from build123d import *

# Parameters (mm, degrees)
SKETCH2_R           = 4.195
SKETCH2_R_2         = 10.305
BOSS_EXTRUDE1_DEPTH = 5.96
FILLET1_R           = 1
SKETCH3_R           = 13.8
SKETCH3_R_2         = 10.305
BOSS_EXTRUDE2_DEPTH = 3.15
FILLET2_R           = 1


with BuildPart() as part:
    # Sketch2 → Boss-Extrude1 (new body)
    with BuildSketch(Plane.XY):
        with BuildLine():
            Line((101.69, 0), (101.69, 15.7))
            ThreePointArc((101.69, 15.7), (97.091576465, 26.801576465), (85.99, 31.4))
            Line((85.99, 31.4), (0, 31.4))
            ThreePointArc((0, 31.4), (-11.101576465, 26.801576465), (-15.7, 15.7))
            ThreePointArc((-15.7, 15.7), (-11.101576465, 4.598423535), (0, 0))
            Line((0, 0), (22.15, 0))
            Line((22.15, 0), (55.695, -63.695))
            ThreePointArc((55.695, -63.695), (58.476021113, -70.408978887), (65.19, -73.19))
            ThreePointArc((65.19, -73.19), (71.903978887, -70.408978887), (74.685, -63.695))
            ThreePointArc((74.685, -63.695), (74.678632674, -63.462256539), (74.673581437, -63.229480796))
            ThreePointArc((74.673581437, -63.229480796), (79.11133413, -43.842864153), (92.1177, -28.7973))
            ThreePointArc((92.1177, -28.7973), (98.886338242, -25.993638242), (101.69, -19.225))
            Line((101.69, -19.225), (101.69, -12.489796776))
            Line((101.69, -12.489796776), (101.69, 0))
        make_face()
        with BuildLine():
            ThreePointArc((69.385, -63.695), (68.156312947, -66.661312947), (65.19, -67.89))
            ThreePointArc((65.19, -67.89), (62.223687053, -60.728687053), (69.385, -63.695))
        make_face(mode=Mode.SUBTRACT)
        with BuildLine():
            ThreePointArc((1.34, 8.01), (-4.097651147, 10.262348853), (-6.35, 15.7))
            ThreePointArc((-6.35, 15.7), (-4.097651147, 21.137651147), (1.34, 23.39))
            Line((1.34, 23.39), (44.31, 23.39))
            ThreePointArc((44.31, 23.39), (52, 15.7), (44.31, 8.01))
            Line((44.31, 8.01), (1.34, 8.01))
        make_face(mode=Mode.SUBTRACT)
        with Locations((92.1177, -19.225)):
            Circle(SKETCH2_R, mode=Mode.SUBTRACT)
        with Locations((85.99, 15.7)):
            Circle(SKETCH2_R_2, mode=Mode.SUBTRACT)
    extrude(amount=BOSS_EXTRUDE1_DEPTH)

    # Fillet1
    fillet1_edges = [part.edges().sort_by_distance(p)[0] for p in [
        (92.1177, -28.7973, 2.98),
        (55.695, -63.695, 2.98),
        (22.15, 0, 2.98),
    ]]
    fillet(fillet1_edges, radius=FILLET1_R)

    # Sketch3 → Boss-Extrude2 (add)
    with BuildSketch(Plane.XY.offset(5.96)):
        with Locations((85.99, 15.7)):
            Circle(SKETCH3_R)
        with Locations((85.99, 15.7)):
            Circle(SKETCH3_R_2, mode=Mode.SUBTRACT)
    extrude(amount=BOSS_EXTRUDE2_DEPTH)

    # Fillet2
    fillet2_edges = [part.edges().sort_by_distance(p)[0] for p in [
        (72.19, 15.7, 9.11),
        (75.685, 15.7, 9.11),
    ]]
    fillet(fillet2_edges, radius=FILLET2_R)


solid = part.part
Source: CAD feature listing. Evaluate the final solid. Frame: model axes, mm. A direction names the side the tool comes from. Give positions to 0.01 mm unless a question says otherwise; leave off trailing zeros. Write each loop counter-clockwise with the first axis right and the second up, starting at its lowest first coordinate (ties: lowest second). Pieces come first, ordered by that corner, then holes. Notation, with made-up numbers: M 80,68.5 L 109,68.5 A18 cw 109,96.5 Z; hole C -20,8 d6. An arc over 180 degrees is marked long. Return JSON: item names as keys, results as strings. Group by question number.
1) First-contact query: pin 1 Ø12 at (x, y) = (59, -50.5) entering from +Z; pin 2 Ø3 at (x, z) = (33.5, 2) entering from -Y; pin 3 Ø1.8 at (x, z) = (7, 3) entering from -Y. Flat tips, straight axial feed; report the tip coordinate or a pass-through.
2) Cut plane B-B, the plane y = -20.5. Output: boundary loops of the cut face in (x, z), then the cut area to 3 significant figures.
3) Set-up query: faces 1 (the face through (11, 0, 3)), 2 (the face through (23, 8.01, 3)), 3 (the face through (93.409, 27.336, 7.02)), 4 (the face through (98.92, -25.96, 2.94)). Return all of +Z, -Z, +X, -X, +Y, -Y with unobstructed straight access to the full face (end or side cutting, diameter ignored); none if empty.
4) Cut plane A-A, the plane x = 18.5. Output: boundary loops of the cut face in (y, z), then the cut area to 3 significant figures.
5) Cut plane C-C, the plane z = 1.75. Give the number of separate pieces and of enclosed holes in the cut face, then the cut area to 3 significant figures.
6) Draft query along Y for faces 5 (the face through (38.775, -31.567, 2.938)), 6 (the face through (55, -9, 0)), 7 (the face through (84.648, 25.917, 3.998)). Return one class per face: released by +Y, released by -Y, zero draft, split by the parting line, or undercut.
7) Ray query, L1, parallel to Z at x = 32, y = 3.5; L2, parallel to Y at x = 31.5, z = 4.75; L3, parallel to Y at x = 44, z = 5.75. Return the intervals inside material, ascending.
8) Cut plane D-D, the plane y = -38.5. Output: boundary loops of the cut face in (x, z).
Data:
{
 "1": {"pin 1": "stops at z = 5.96", "pin 2": "stops at y = -24.4", "pin 3": "stops at y = 0"},
 "2": {"outline": "M 32.95,0 L 88.12,0 L 88.12,5.96 L 32.95,5.96 Z; M 96.11,0 L 101.6,0 L 101.6,5.96 L 96.11,5.96 Z", "area": "362 mm²"},
 "3": {"face 1": "+Z, -Z, -X, -Y", "face 2": "+Z, -Z", "face 3": "+Z", "face 4": "+Z, -Z, +X, -Y"},
 "4": {"outline": "M 0,0 L 8.01,0 L 8.01,5.96 L 0,5.96 Z; M 23.39,0 L 31.4,0 L 31.4,5.96 L 23.39,5.96 Z", "area": "95.5 mm²"},
 "5": {"separate pieces": "1", "enclosed holes": "4", "area": "5,590 mm²"},
 "6": {"face 5": "released by -Y", "face 6": "zero draft", "face 7": "undercut"},
 "7": {"L1": "z = 0 to 5.96", "L2": "y = -17.75 to 8.01, 23.39 to 31.4", "L3": "y = -41.49 to 8.01, 23.39 to 31.4"},
 "8": {"outline": "M 42.43,0 L 82.35,0 L 82.35,5.96 L 42.43,5.96 Z"}
}
